from build123d import *

# Parameters (mm, degrees)
SKETCH1_W               = 190.5
SKETCH1_H               = 6.35
BOSS_EXTRUDE1_DEPTH     = 12.7
SKETCH2_W               = 25.4
SKETCH2_H               = 6.35
BOSS_EXTRUDE2_DEPTH     = 6.35
LPATTERN1_COUNT         = 3
LPATTERN1_PITCH         = 50.8
MIRROR1_COPY_1_SKETCH_W = 25.4
MIRROR1_COPY_1_SKETCH_H = 6.35
MIRROR1_COPY_1_DEPTH    = 6.35
MIRROR1_COPY_2_SKETCH_W = 25.4
MIRROR1_COPY_2_SKETCH_H = 6.35
MIRROR1_COPY_2_DEPTH    = 6.35


with BuildPart() as part:
    # Sketch1 → Boss-Extrude1 (new body)
    with BuildSketch(Plane.XY):
        with Locations((-30.030526088, -11.1125)):
            Rectangle(SKETCH1_W, SKETCH1_H)
    extrude(amount=BOSS_EXTRUDE1_DEPTH)

    # Sketch2 → Boss-Extrude2 (add)
    with BuildSketch(Plane(origin=(0, 0, 0), x_dir=(-1, 0, 0), z_dir=(0, 0, -1))):
        with Locations((87.180526088, -11.1125)):
            Rectangle(SKETCH2_W, SKETCH2_H)
    boss_extrude2 = extrude(amount=BOSS_EXTRUDE2_DEPTH)

    # LPattern1: Boss-Extrude2 ×3
    with Locations(*[(i * LPATTERN1_PITCH, 0, 0) for i in range(1, LPATTERN1_COUNT)]):
        add(boss_extrude2)

    # Mirror1: Boss-Extrude2 across plane
    add(boss_extrude2.mirror(Plane(origin=(-125.280526088, -20.6375, 6.35), x_dir=(1, 0, 0), z_dir=(0, 0, 1))))

    # Mirror1 copy 1 sketch → Mirror1 copy 1 (add)
    with BuildSketch(Plane(origin=(50.8, 0, 12.7), x_dir=(-1, 0, 0), z_dir=(0, 0, 1))):
        with Locations((87.180526088, 11.1125)):
            Rectangle(MIRROR1_COPY_1_SKETCH_W, MIRROR1_COPY_1_SKETCH_H)
    extrude(amount=MIRROR1_COPY_1_DEPTH)

    # Mirror1 copy 2 sketch → Mirror1 copy 2 (add)
    with BuildSketch(Plane(origin=(101.6, 0, 12.7), x_dir=(-1, 0, 0), z_dir=(0, 0, 1))):
        with Locations((87.180526088, 11.1125)):
            Rectangle(MIRROR1_COPY_2_SKETCH_W, MIRROR1_COPY_2_SKETCH_H)
    extrude(amount=MIRROR1_COPY_2_DEPTH)


solid = part.part
Part model, mm, in its own coordinate system. A direction names the side the tool comes from. Give positions to 0.01 mm unless a question says otherwise; leave off trailing zeros. Loops run counter-clockwise (first coordinate to the right, second up) from the corner with the lowest first, then second, coordinate; pieces in that order, holes last. Notation, with made-up numbers: (44.25, 14.5) -> (92.25, 14.5) arc R29 ccw to (92.25, 42.5) -> close; hole circle Ø6 at (52, 13). An arc over 180 degrees is marked (long way). Write each question's results on one line, items separated by ' | '. Start each with the question number.
Q1. Band-saw the part on C-C on x = -64.5. List the corners of the cut face in (y, z).
Q2. Pull direction X, two halves, no side cores. Call faces 1 (the face through (1.719, -11, 16)), 2 (the face through (15, -11, -6.35)), 3 (the face through (-99.881, -11, -3)), 4 (the face through (-74.481, -11, -3)): +X half, -X half, draft (parallel to the pull), parting line (faces both ways), or undercut.
Q3. Wall check: L1, parallel to X at y = -10.75, z = 17.5; L2, parallel to Z at x = 42.5, y = -10. Give the ranges that are in metal, low to high.
Q4. Band-saw the part on A-A on z = -2.25. List the corners of the cut face in (x, y).
Q5. Which spindle directions (+Z, -Z, +X, -X, +Y, -Y) get a long thin tool onto all of the face, cutting with end or side? Do faces 5 (the face through (27.119, -11, 16)), 6 (the face through (1.719, -11, -3)), 7 (the face through (-49.081, -11, 16)). Say none if no direction does.
Q6. Band-saw the part on B-B on y = -12. List the corners of the cut face in (x, z), plus the area to 3 significant figures.
Q7. Pin check, flat tips, straight feed: P1, Ø1.9, axis at y = -9.5, z = -4, coming from the +X side; P2, Ø3, axis at x = 53, y = -10.5, coming from the -Z side; P3, Ø3, axis at y = -10.5, z = -2.5, coming from the -X side. Stop position of each tip, or through.
Results are:
1) outline: (-14.29, 0) -> (-7.94, 0) -> (-7.94, 12.7) -> (-14.29, 12.7) -> close
2) face 1: undercut | face 2: draft | face 3: -X half | face 4: undercut
3) L1: x = -99.88 to -74.48, -49.08 to -23.68, 1.72 to 27.12 | L2: z = 0 to 12.7
4) outline: (-99.88, -14.29) -> (-74.48, -14.29) -> (-74.48, -7.94) -> (-99.88, -7.94) -> close; (-49.08, -14.29) -> (-23.68, -14.29) -> (-23.68, -7.94) -> (-49.08, -7.94) -> close; (1.72, -14.29) -> (27.12, -14.29) -> (27.12, -7.94) -> (1.72, -7.94) -> close
5) face 5: +Z, +X, +Y, -Y | face 6: -Z, +Y, -Y | face 7: +Z, +Y, -Y
6) outline: (-125.28, 0) -> (-99.88, 0) -> (-99.88, -6.35) -> (-74.48, -6.35) -> (-74.48, 0) -> (-49.08, 0) -> (-49.08, -6.35) -> (-23.68, -6.35) -> (-23.68, 0) -> (1.72, 0) -> (1.72, -6.35) -> (27.12, -6.35) -> (27.12, 0) -> (65.22, 0) -> (65.22, 12.7) -> (27.12, 12.7) -> (27.12, 19.05) -> (1.72, 19.05) -> (1.72, 12.7) -> (-23.68, 12.7) -> (-23.68, 19.05) -> (-49.08, 19.05) -> (-49.08, 12.7) -> (-74.48, 12.7) -> (-74.48, 19.05) -> (-99.88, 19.05) -> (-99.88, 12.7) -> (-125.28, 12.7) -> close | area: 3,390 mm²
7) P1: stops at x = 27.12 | P2: stops at z = 0 | P3: stops at x = -99.88
